```python
from build123d import *

# Parameters (mm, degrees)
SKETCH_1_W               = 94
SKETCH_1_H               = 94
EXTRUDE_1_DEPTH          = 80
SKETCH_1_3_W             = 90
SKETCH_1_3_H             = 90
CUT_EXTRUDE_1_DEPTH      = 78
SKETCH_1_5_W             = 124
SKETCH_1_5_H             = 124
SKETCH_1_5_W_2           = 94
SKETCH_1_5_H_2           = 94
EXTRUDE_2_DEPTH          = 2
FILLET_1_R               = 2
CUT_EXTRUDE_4_DEPTH      = 162.89480683
CUT_EXTRUDE_5_DEPTH      = 162.89480683
CUT_EXTRUDE_6_DEPTH      = 162.89480683
SKETCH_6_W               = 13.428571429
SKETCH_6_H               = 76.0093606
CUT_EXTRUDE_7_DEPTH      = 150.641361191
SKETCH_6_3_W             = 13.428571429
SKETCH_6_3_H             = 76.0093606
CUT_EXTRUDE_8_DEPTH      = 150.641361191
CUT_EXTRUDE_9_DEPTH      = 150.641361191
CUT_EXTRUDE_9_DEPTH_BACK = 150.641361191
SKETCH_6_4_W             = 13.428571428
SKETCH_6_4_H             = 76.0093606
SKETCH_8_R               = 2.5
CUT_EXTRUDE_13_DEPTH     = 135.627134923
SKETCH_8_4_R             = 8
CUT_EXTRUDE_16_DEPTH     = 1
SKETCH_8_5_R             = 10
CUT_EXTRUDE_17_DEPTH     = 135.627134923
FILLET_2_R               = 2
FILLET_4_R               = 2
FILLET_10_R              = 1
SKETCH_10_R              = 1.7
CUT_EXTRUDE_18_DEPTH     = 10


with BuildPart() as part:
    # 草图1 → 凸台-拉伸1 (new body)
    with BuildSketch(Plane(origin=(0, 0, 0), x_dir=(1, 0, 0), z_dir=(0, 1, 0))):
        with Locations((2.121267759, 27.044530874)):
            Rectangle(SKETCH_1_W, SKETCH_1_H)
    extrude(amount=-EXTRUDE_1_DEPTH)

    # 草图1<3> → 切除-拉伸1 (cut)
    with BuildSketch(Plane(origin=(0, 0, 0), x_dir=(1, 0, 0), z_dir=(0, 1, 0))):
        with Locations((2.121267759, 27.044530874)):
            Rectangle(SKETCH_1_3_W, SKETCH_1_3_H)
    extrude(amount=-CUT_EXTRUDE_1_DEPTH, mode=Mode.SUBTRACT)

    # 草图1<5> → 凸台-拉伸2 (add)
    with BuildSketch(Plane(origin=(0, 0, 0), x_dir=(1, 0, 0), z_dir=(0, 1, 0))):
        with Locations((2.121267759, 27.044530874)):
            Rectangle(SKETCH_1_5_W, SKETCH_1_5_H)
        with Locations((2.121267759, 27.044530874)):
            Rectangle(SKETCH_1_5_W_2, SKETCH_1_5_H_2, mode=Mode.SUBTRACT)
    extrude(amount=-EXTRUDE_2_DEPTH)

    # 圆角1
    fillet_1_edges = [part.edges().sort_by_distance(p)[0] for p in [
        (2.121267759, 0, -72.044530874),
        (47.121267759, 0, -27.044530874),
        (-42.878732241, 0, -27.044530874),
        (2.121267759, 0, 17.955469126),
    ]]
    fillet(fillet_1_edges, radius=FILLET_1_R)

    # 草图5 → 切除-拉伸4 (cut, through all)
    with BuildSketch(Plane(origin=(49.121267759, 0, 0), x_dir=(0, 0, -1), z_dir=(1, 0, 0))):
        Polygon((-6.526897697, -78.001337229), (-6.526897697, -2), (6.901673731, -2), (6.901673731, -78.002674457), align=None)
    extrude(amount=-CUT_EXTRUDE_4_DEPTH, mode=Mode.SUBTRACT)

    # 草图5<5> → 切除-拉伸5 (cut, through all)
    with BuildSketch(Plane(origin=(49.121267759, 0, 0), x_dir=(0, 0, -1), z_dir=(1, 0, 0))):
        Polygon((20.33024516, -78.004011686), (20.33024516, -2), (33.758816589, -2), (33.758816589, -78.005348914), align=None)
    extrude(amount=-CUT_EXTRUDE_5_DEPTH, mode=Mode.SUBTRACT)

    # 草图5<6> → 切除-拉伸6 (cut, through all)
    with BuildSketch(Plane(origin=(49.121267759, 0, 0), x_dir=(0, 0, -1), z_dir=(1, 0, 0))):
        Polygon((47.187388017, -78.006686143), (47.187388017, -2), (60.615959446, -2), (60.615959446, -78.008023372), align=None)
    extrude(amount=-CUT_EXTRUDE_6_DEPTH, mode=Mode.SUBTRACT)

    # 草图6 → 切除-拉伸7 (cut, through all)
    with BuildSketch(Plane(origin=(0, 0, -74.044530874), x_dir=(-1, 0, 0), z_dir=(0, 0, -1))):
        with Locations((-28.978410616, -40.0046803)):
            Rectangle(SKETCH_6_W, SKETCH_6_H)
    extrude(amount=-CUT_EXTRUDE_7_DEPTH, mode=Mode.SUBTRACT)

    # 草图6<3> → 切除-拉伸8 (cut, through all)
    with BuildSketch(Plane(origin=(0, 0, -74.044530874), x_dir=(-1, 0, 0), z_dir=(0, 0, -1))):
        with Locations((-2.12126776, -40.0046803)):
            Rectangle(SKETCH_6_3_W, SKETCH_6_3_H)
    extrude(amount=-CUT_EXTRUDE_8_DEPTH, mode=Mode.SUBTRACT)

    # 草图6<4> → 切除-拉伸9 (cut, two sides: drawn at the far end of the back side and taken through both)
    with BuildSketch(Plane(origin=(0, 0, -74.044530874), x_dir=(-1, 0, 0), z_dir=(0, 0, -1)).offset(-CUT_EXTRUDE_9_DEPTH_BACK)):
        with Locations((24.735875098, -40.0046803)):
            Rectangle(SKETCH_6_4_W, SKETCH_6_4_H)
    extrude(amount=CUT_EXTRUDE_9_DEPTH + CUT_EXTRUDE_9_DEPTH_BACK, mode=Mode.SUBTRACT)

    # 草图8 → 切除-拉伸13 (cut, through all)
    with BuildSketch(Plane(origin=(0, -78, 0), x_dir=(-1, 0, 0), z_dir=(0, -1, 0))):
        with Locations(Location((-2.148108933, 27.017689701, 0), (0, 0, 270))):
            Circle(SKETCH_8_R)
    extrude(amount=CUT_EXTRUDE_13_DEPTH, mode=Mode.SUBTRACT)

    # 草图8<4> → 切除-拉伸16 (cut)
    with BuildSketch(Plane(origin=(0, -78, 0), x_dir=(-1, 0, 0), z_dir=(0, -1, 0))):
        with Locations(Location((-2.148108933, 27.017689701, 0), (0, 0, 213.287140052))):
            Circle(SKETCH_8_4_R)
    extrude(amount=CUT_EXTRUDE_16_DEPTH, mode=Mode.SUBTRACT)

    # 草图8<5> → 切除-拉伸17 (cut, through all)
    with BuildSketch(Plane(origin=(0, -78, 0), x_dir=(-1, 0, 0), z_dir=(0, -1, 0))):
        with Locations(Location((20.365311654, 4.531110288, 0), (0, 0, 256.445379393))):
            Circle(SKETCH_8_5_R)
        with Locations(Location((-24.634688346, 49.531110288, 0), (0, 0, 283.712868299))):
            Circle(SKETCH_8_5_R)
        with Locations(Location((-24.634688346, 4.531110288, 0), (0, 0, 283.712868299))):
            Circle(SKETCH_8_5_R)
        with Locations(Location((20.365311654, 49.531110288, 0), (0, 0, 256.445379393))):
            Circle(SKETCH_8_5_R)
    extrude(amount=CUT_EXTRUDE_17_DEPTH, mode=Mode.SUBTRACT)

    # 圆角2
    fillet_2_edges = [part.edges().sort_by_distance(p)[0] for p in [
        (-59.878732241, -1, 34.955469126),
        (-59.878732241, -1, -89.044530874),
        (64.121267759, -1, -89.044530874),
        (64.121267759, -1, 34.955469126),
    ]]
    fillet(fillet_2_edges, radius=FILLET_2_R)

    # 圆角4
    fillet_4_edges = [part.edges().sort_by_distance(p)[0] for p in [
        (2.121267759, 0, 34.955469126),
        (-59.878732241, 0, -27.044530874),
        (64.121267759, 0, -27.044530874),
        (2.121267759, 0, -89.044530874),
        (-59.292945803, 0, -88.458744437),
        (63.535481322, 0, -88.458744437),
        (-59.292945803, 0, 34.369682688),
        (63.535481322, 0, 34.369682688),
    ]]
    fillet(fillet_4_edges, radius=FILLET_4_R - 0.0001)  # a hair under: the kernel refuses the full size

    # 圆角10
    fillet_10_edges = [part.edges().sort_by_distance(p)[0] for p in [
        (2.121267759, -80, 19.955469126),
        (-44.878732241, -80, -27.044530874),
        (2.121267759, -80, -74.044530874),
        (49.121267759, -80, -27.044530874),
    ]]
    fillet(fillet_10_edges, radius=FILLET_10_R)

    # 草图10 → 切除-拉伸18 (cut)
    with BuildSketch(Plane.XZ.offset(7)):
        with Locations(Location((60.121267759, 29.955469126, 0), (0, 0, 270))):
            Circle(SKETCH_10_R)
        with Locations(Location((60.121267759, -85.044530874, 0), (0, 0, 270))):
            Circle(SKETCH_10_R)
        with Locations(Location((-54.878732241, -85.044530874, 0), (0, 0, 270))):
            Circle(SKETCH_10_R)
        with Locations(Location((-54.878732241, 29.955469126, 0), (0, 0, 270))):
            Circle(SKETCH_10_R)
    extrude(amount=-CUT_EXTRUDE_18_DEPTH, mode=Mode.SUBTRACT)


solid = part.part
```
Geometry: final body of the model. Coordinates: model frame, mm. A direction names the side the tool comes from. Coordinates: 2 decimals unless noted, no trailing zeros. Write item = value, one per line.
(1) Pull-direction query (X, two-part tool) for faces 5 (the flat face through (47.121, -39, -66)), 6 (the flat face through (12, -40, -74.045)), 7 (the cylindrical face through (-10.66, -78.99, -2.12)), 8 (the flat face through (-44.879, -40, -37)); classes: pulls with the +X half, pulls with the -X half, needs draft (parallel to the pull), parting line crosses it, or undercut.
Solved:
face_5 = undercut
face_6 = needs draft
face_7 = undercut
face_8 = pulls with the -X half
(2) Pin query (flat end, axial travel): pin 1 Ø9 at (y, z) = (-27, -68.5) entering from -X; pin 2 Ø10.5 at (x, y) = (-40.5, -36.5) entering from +Z; pin 3 Ø10 at (x, z) = (29.5, -4) entering from +Y; pin 4 Ø3.5 at (x, z) = (39.5, -43.5) entering from +Y. Return the tip coordinate at first contact, or that it passes through.
Solved:
pin_1 = -44.88
pin_2 = 19.96
pin_3 = through
pin_4 = -78
(3) Access query for faces 1 (the cylindrical face through (60.632, -1.014, -86.666)), 2 (the flat face through (47.121, -39, -40)), 3 (the flat face through (22.264, -40, -73)), 4 (the flat face through (48, -40, -60.616)). Directions: +Z, -Z, +X, -X, +Y, -Y. A direction counts if a zero-diameter tool reaches every point of the face in a straight line with its end or side. Return the directions, or none.
Solved:
face_1 = +Y, -Y
face_2 = +Y
face_3 = +Z, -Z
face_4 = +X, -X
(4) Cut plane B-B on z = -27.5. Count the separate pieces of the cut face and the enclosed holes in it, plus the area to 3 significant figures.
Solved:
separate_pieces = 4
enclosed_holes = 0
area = 231 mm²
(5) Line query: line 1 (Z direction, x = 46.5, y = -31); line 2 (X direction, y = -61, z = 9); line 3 (Y direction, x = 55.5, z = -73.5). Output: solid intervals per line, ascending.
Solved:
line_1 = -74.04 to -72.04, 17.96 to 19.96
line_2 = -44.88 to -42.88, 47.12 to 49.12
line_3 = -2 to 0
